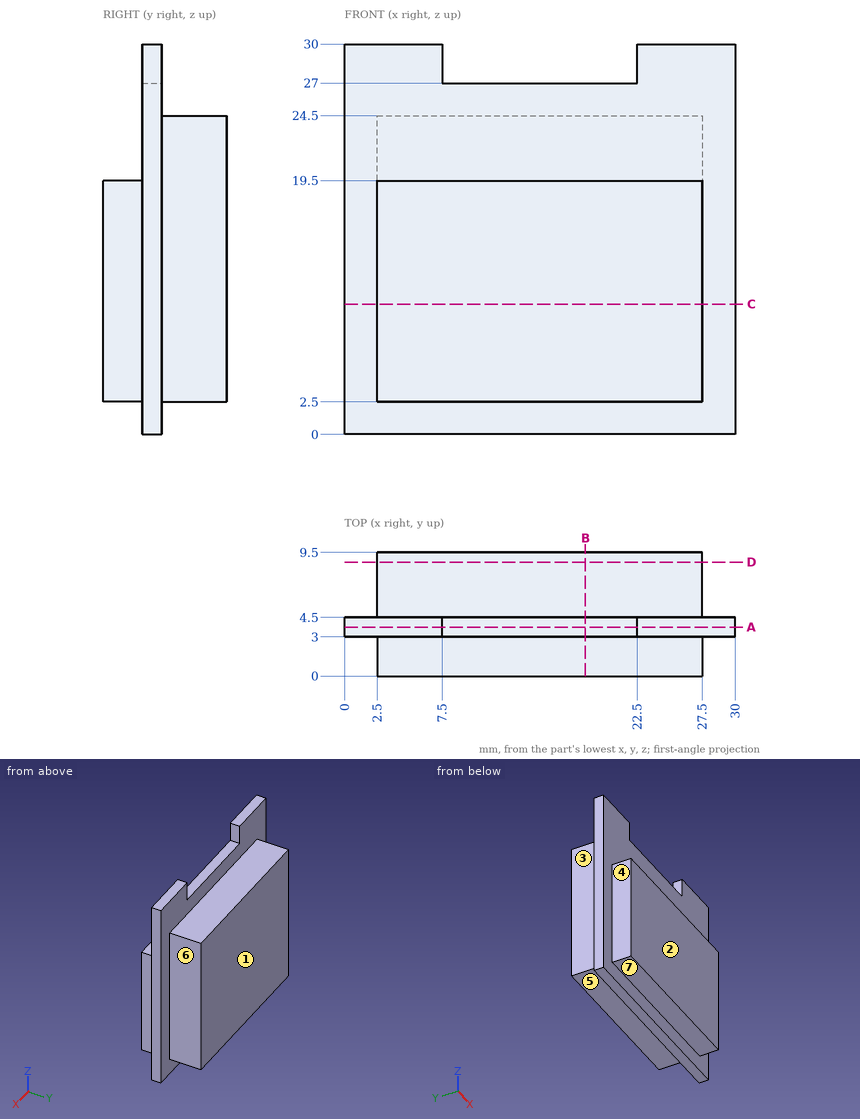
For this review, use the dimensioned drawing (mm, ordinates from the lowest corner) and the shaded views. A direction names the side the tool comes from. Coordinates: 2 decimals unless noted, no trailing zeros. Write each loop counter-clockwise with the first axis right and the second up, starting at its lowest first coordinate (ties: lowest second). Pieces come first, ordered by that corner, then holes. Notation, with made-up numbers: (88.25, 89) -> (116.25, 89) arc R24 ccw to (116.25, 110) -> close; hole circle Ø8 at (56.5, 88). An arc over 180 degrees is marked (long way). Write each question's results on one line, items separated by ' | '. Start each with the question number.
(1) Take a section at A-A on y = 3.75. Write out the cut boundary in (x, z), and give its area (3 significant figures).
(2) Take a section at C-C on z = 10. Write out the cut boundary in (x, y).
(3) Take a section at B-B on x = 18.5. Write out the cut boundary in (y, z).
(4) Take a section at D-D on y = 8.75. Write out the cut boundary in (x, z).
(5) Clearance check with flat-ended pins moving along their axes: P1, Ø2, axis at x = 16.5, y = 6, coming from the +Z side; P2, Ø1.5, axis at x = 19, y = 7.5, coming from the -Z side; P3, Ø2.5, axis at y = 1.5, z = 7.5, coming from the -X side; P4, Ø1.2, axis at y = 4, z = 28, coming from the -X side. State where each tip first meets the part, or that it passes through.
(6) For line 1 along X through (y, z) = (2.5, 18); line 2 along Z through (x, y) = (5.5, 8.5); line 3 along Y through (x, z) = (18.5, 24.75), list the stretches that pass through material, from the lowest coordinate up. Write a range as from..to.
(7) Tool access review of the marked faces 4, 5, 6 and 7: name each direction out of +Z, -Z, +X, -X, +Y, -Y from which nothing blocks a thin tool from reaching the whole face with its end or side.
(8) The part is to be moulded in two halves that separate along Y. For the marked faces 1, 2 and 3, say which applies: pulls with the +Y half, pulls with the -Y half, needs draft (parallel to the pull), parting line crosses it, or undercut.
Results found:
1) outline: (0, 0) -> (30, 0) -> (30, 30) -> (22.5, 30) -> (22.5, 27) -> (7.5, 27) -> (7.5, 30) -> (0, 30) -> close | area: 855 mm2
2) outline: (0, 3) -> (2.5, 3) -> (2.5, 0) -> (27.5, 0) -> (27.5, 3) -> (30, 3) -> (30, 4.5) -> (27.5, 4.5) -> (27.5, 9.5) -> (2.5, 9.5) -> (2.5, 4.5) -> (0, 4.5) -> close
3) outline: (0, 2.5) -> (3, 2.5) -> (3, 0) -> (4.5, 0) -> (4.5, 2.5) -> (9.5, 2.5) -> (9.5, 24.5) -> (4.5, 24.5) -> (4.5, 27) -> (3, 27) -> (3, 19.5) -> (0, 19.5) -> close
4) outline: (2.5, 2.5) -> (27.5, 2.5) -> (27.5, 24.5) -> (2.5, 24.5) -> close
5) P1: stops at z = 24.5 | P2: stops at z = 2.5 | P3: stops at x = 2.5 | P4: stops at x = 0
6) line 1: x = 2.5..27.5 | line 2: z = 2.5..24.5 | line 3: y = 3..4.5
7) face 4: +Z, -Z, -X, -Y | face 5: -Z, +X, -X, +Y | face 6: +Z, -Z, +X, +Y | face 7: -Z, +X, -X, -Y
8) face 1: pulls with the +Y half | face 2: pulls with the -Y half | face 3: needs draft
